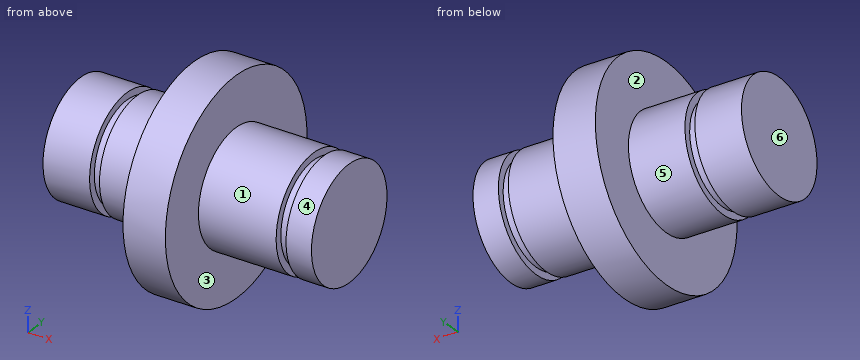
```python
from build123d import *

# Parameters (mm, degrees)
SCHIZZO1_R                   = 7.5
ESTRUSIONE_ESTRUSIONE1_DEPTH = 9.5
SCHIZZO3_R                   = 7.5
SCHIZZO3_R_2                 = 4
TAGLIO_ESTRUSIONE1_DEPTH     = 8
TAGLIO_ESTRUSIONE2_START     = -8
SCHIZZO5_R                   = 7.5
SCHIZZO5_R_2                 = 4
TAGLIO_ESTRUSIONE2_DEPTH     = 8
SCHIZZO4_W                   = 0.7
SCHIZZO4_H                   = 0.5


with BuildPart() as part:
    # Schizzo1 → Estrusione-Estrusione1 (new, symmetric)
    with BuildSketch(Plane(origin=(0, 0, 0), x_dir=(0, 0, -1), z_dir=(1, 0, 0))):
        Circle(SCHIZZO1_R)
    extrude(amount=ESTRUSIONE_ESTRUSIONE1_DEPTH, both=True)

    # Schizzo3 → Taglio-Estrusione1 (cut)
    with BuildSketch(Plane(origin=(9.5, 0, 0), x_dir=(0, 0, -1), z_dir=(1, 0, 0))):
        Circle(SCHIZZO3_R)
        Circle(SCHIZZO3_R_2, mode=Mode.SUBTRACT)
    extrude(amount=-TAGLIO_ESTRUSIONE1_DEPTH, mode=Mode.SUBTRACT)

    # Schizzo5 → Taglio-Estrusione2 (cut)
    with BuildSketch(Plane.ZY.offset(9.5).offset(TAGLIO_ESTRUSIONE2_START)):
        Circle(SCHIZZO5_R)
        with Locations(Location((0, 0, 0), (0, 0, 180))):
            Circle(SCHIZZO5_R_2, mode=Mode.SUBTRACT)
    extrude(amount=TAGLIO_ESTRUSIONE2_DEPTH, mode=Mode.SUBTRACT)

    # Schizzo4 → Taglia-Rivoluzione1 (revolve, cut)
    with BuildSketch(Plane.XY, mode=Mode.PRIVATE) as taglia_rivoluzione1_sk:
        with Locations((7.35, 3.75)):
            Rectangle(SCHIZZO4_W, SCHIZZO4_H)
        with Locations((-5.85, 3.75)):
            Rectangle(SCHIZZO4_W, SCHIZZO4_H)
    revolve(taglia_rivoluzione1_sk.sketch.rotate(Axis((0, 0, 0), (-1, 0, 0)), 90), axis=Axis((0, 0, 0), (-1, 0, 0)), mode=Mode.SUBTRACT)


solid = part.part
```
Input: part model. Units: mm. Frame: model coordinates. Face numbers are marked on the shaded views. A direction names the side the tool comes from. Coordinates: 2 decimals unless noted, no trailing zeros. Write each loop counter-clockwise with the first axis right and the second up, starting at its lowest first coordinate (ties: lowest second). Pieces come first, ordered by that corner, then holes. Notation, with made-up numbers: (76, 78.5) - (121, 78.5) arc R11 cw to (121, 90.5) - close; hole circle Ø1 at (-22.75, 23). An arc over 180 degrees is marked (long way). Put each result on its own line as item: value. Start each with the question number.
1) Cut plane D-D (z = -6). Return the cut outline in (x, y).
2) Reachability of the marked faces 4, 5 and 6 from +Z, -Z, +X, -X, +Y, -Y: full face, straight path, thin tool, end or side. Return the list, or none.
3) Cut plane A-A (y = 0). Return the cut outline in (x, z), plus the area to 3 significant figures.
4) Mould query, pull axis X, two halves, no side actions, for the marked faces 1, 2 and 3. Classes: pulls with the +X half, pulls with the -X half, needs draft (parallel to the pull), parting line crosses it, or undercut.
5) Contact query for flat-ended pins moving along their axis: pin 1 (4 mm diameter, centred on x = 4.5, y = -5.5, fed in from -Z); pin 2 (6 mm diameter, centred on x = -0.5, y = 4, fed in from -Z); pin 3 (1 mm diameter, centred on y = 4.5, z = -5.5, fed in from +X). Output: stop coordinate, or through.
6) Ray query, L1, parallel to X at y = 3.25, z = -2.5; L2, parallel to Y at x = 0, z = 0.25; L3, parallel to Z at x = -3.25, y = -1.75. Return the intervals inside material, ascending.
7) Cut plane C-C (x = 5). Return the cut outline in (y, z), plus the area to 3 significant figures.
Resolved:
1. outline: (-1.5, -4.5) - (1.5, -4.5) - (1.5, 4.5) - (-1.5, 4.5) - close
2. face 4: +X
2. face 5: -X
2. face 6: +Z, -Z, -X, +Y, -Y
3. outline: (-9.5, -4) - (-6.2, -4) - (-6.2, -3.5) - (-5.5, -3.5) - (-5.5, -4) - (-1.5, -4) - (-1.5, -7.5) - (1.5, -7.5) - (1.5, -4) - (7, -4) - (7, -3.5) - (7.7, -3.5) - (7.7, -4) - (9.5, -4) - (9.5, 4) - (7.7, 4) - (7.7, 3.5) - (7, 3.5) - (7, 4) - (1.5, 4) - (1.5, 7.5) - (-1.5, 7.5) - (-1.5, 4) - (-5.5, 4) - (-5.5, 3.5) - (-6.2, 3.5) - (-6.2, 4) - (-9.5, 4) - close
3. area: 172 mm2
4. face 1: needs draft
4. face 2: pulls with the -X half
4. face 3: pulls with the +X half
5. pin 1: stops at z = -1.94
5. pin 2: stops at z = -7.43
5. pin 3: stops at x = 1.5
6. L1: x = -1.5 to 1.5
6. L2: y = -7.5 to 7.5
6. L3: z = -3.6 to 3.6
7. outline: circle Ø8 at (0, 0)
7. area: 50.3 mm2
